```python
from build123d import *

# Parameters (mm, degrees)
SKETCH_1_W          = 63
SKETCH_1_H          = 15
SKETCH_1_R          = 1.1
SKETCH_1_R_2        = 1
SKETCH_1_R_3        = 1.5
SKETCH_1_R_4        = 2.6
EXTRUDE_1_DEPTH     = 2
SKETCH_2_R          = 1.4
EXTRUDE_2_DEPTH     = 2
SKETCH_3_R          = 3
CUT_EXTRUDE_1_DEPTH = 1.5
SKETCH_4_W          = 46
SKETCH_4_H          = 1.5
EXTRUDE_3_DEPTH     = 5
SKETCH_2_3_R        = 0.95
CUT_EXTRUDE_2_DEPTH = 1.5
CUT_EXTRUDE_3_DEPTH = 0.25
SKETCH_1_7_W        = 15
SKETCH_1_7_H        = 15
SKETCH_1_7_R        = 1.5
SKETCH_1_7_R_2      = 1.1
EXTRUDE_4_DEPTH     = 4
SKETCH_1_8_R        = 6
SKETCH_1_8_R_2      = 1.5
SKETCH_1_8_R_3      = 1.1
CUT_EXTRUDE_4_DEPTH = 2
CUT_EXTRUDE_5_DEPTH = 15
SKETCH_1_9_R        = 4
SKETCH_1_9_R_2      = 2.6
EXTRUDE_5_DEPTH     = 4


with BuildPart() as part:
    # 草图1 → 凸台-拉伸1 (new body)
    with BuildSketch(Plane(origin=(0, 0, 0), x_dir=(1, 0, 0), z_dir=(0, 1, 0))):
        Rectangle(SKETCH_1_W, SKETCH_1_H)
        with Locations(Location((-12.830127019, -2.5, 0), (0, 0, 270))):
            Circle(SKETCH_1_R, mode=Mode.SUBTRACT)
        with Locations(Location((3, 0, 0), (0, 0, 270))):
            Circle(SKETCH_1_R_2, mode=Mode.SUBTRACT)
        with Locations(Location((13, 0, 0), (0, 0, 270))):
            Circle(SKETCH_1_R_2, mode=Mode.SUBTRACT)
        with Locations(Location((-8.5, 0, 0), (0, 0, 270))):
            Circle(SKETCH_1_R_3, mode=Mode.SUBTRACT)
        with Locations(Location((-4.169872981, 2.5, 0), (0, 0, 270))):
            Circle(SKETCH_1_R, mode=Mode.SUBTRACT)
        with Locations(Location((8, 5, 0), (0, 0, 270))):
            Circle(SKETCH_1_R_2, mode=Mode.SUBTRACT)
        with Locations(Location((8, 0, 0), (0, 0, 270))):
            Circle(SKETCH_1_R_4, mode=Mode.SUBTRACT)
        with Locations(Location((24, 3.5, 0), (0, 0, 270))):
            Circle(SKETCH_1_R, mode=Mode.SUBTRACT)
        with Locations(Location((24, -3.5, 0), (0, 0, 270))):
            Circle(SKETCH_1_R, mode=Mode.SUBTRACT)
        with Locations(Location((20.5, 0, 0), (0, 0, 270))):
            Circle(SKETCH_1_R, mode=Mode.SUBTRACT)
        with Locations(Location((24, 0, 0), (0, 0, 270))):
            Circle(SKETCH_1_R_3, mode=Mode.SUBTRACT)
        with Locations(Location((27.5, 0, 0), (0, 0, 270))):
            Circle(SKETCH_1_R, mode=Mode.SUBTRACT)
    extrude(amount=EXTRUDE_1_DEPTH)

    # 草图2 → 凸台-拉伸2 (add)
    with BuildSketch(Plane.XY.offset(7.5)):
        with Locations(Location((-23.5, 0.6, 0), (0, 0, 205.376933525))):
            Circle(SKETCH_2_R)
        with Locations(Location((-8.5, 0.6, 0), (0, 0, 205.376933525))):
            Circle(SKETCH_2_R)
        with Locations(Location((6.5, 0.6, 0), (0, 0, 205.376933525))):
            Circle(SKETCH_2_R)
    extrude(amount=EXTRUDE_2_DEPTH)

    # 草图3 → 切除-拉伸1 (cut)
    with BuildSketch(Plane.XZ):
        with Locations(Location((-8.5, 0, 0), (0, 0, 270))):
            Circle(SKETCH_3_R)
    extrude(amount=-CUT_EXTRUDE_1_DEPTH, mode=Mode.SUBTRACT)

    # 草图4 → 凸台-拉伸3 (add)
    with BuildSketch(Plane.XZ):
        with Locations((-8.5, 6.75)):
            Rectangle(SKETCH_4_W, SKETCH_4_H)
    extrude(amount=EXTRUDE_3_DEPTH)

    # 草图2<3> → 切除-拉伸2 (cut)
    with BuildSketch(Plane.XY.offset(7.5)):
        with Locations((-23.5, -3.4)):
            Circle(SKETCH_2_3_R)
        with Locations((-8.5, -3.4)):
            Circle(SKETCH_2_3_R)
        with Locations((6.5, -3.4)):
            Circle(SKETCH_2_3_R)
    extrude(amount=-CUT_EXTRUDE_2_DEPTH, mode=Mode.SUBTRACT)

    # 草图5 → 切除-拉伸3 (cut)
    with BuildSketch(Plane(origin=(0, 0, 6), x_dir=(-1, 0, 0), z_dir=(0, 0, -1))):
        Polygon((22.403034489, -1.5), (24.596965511, -1.5), (25.693931023, -3.4), (24.596965511, -5.3), (22.403034489, -5.3), (21.306068977, -3.4), align=None)
        Polygon((6.306068977, -3.4), (7.403034489, -1.5), (9.596965511, -1.5), (10.693931023, -3.4), (9.596965511, -5.3), (7.403034489, -5.3), align=None)
        Polygon((-8.693931023, -3.4), (-7.596965511, -1.5), (-5.403034489, -1.5), (-4.306068977, -3.4), (-5.403034489, -5.3), (-7.596965511, -5.3), align=None)
    extrude(amount=-CUT_EXTRUDE_3_DEPTH, mode=Mode.SUBTRACT)

    # 草图1<7> → 凸台-拉伸4 (add)
    with BuildSketch(Plane(origin=(0, 0, 0), x_dir=(1, 0, 0), z_dir=(0, 1, 0))):
        with Locations((24, 0)):
            Rectangle(SKETCH_1_7_W, SKETCH_1_7_H)
        with Locations(Location((24, 0, 0), (0, 0, 270))):
            Circle(SKETCH_1_7_R, mode=Mode.SUBTRACT)
        with Locations(Location((27.5, 0, 0), (0, 0, 270))):
            Circle(SKETCH_1_7_R_2, mode=Mode.SUBTRACT)
        with Locations(Location((24, -3.5, 0), (0, 0, 270))):
            Circle(SKETCH_1_7_R_2, mode=Mode.SUBTRACT)
        with Locations(Location((20.5, 0, 0), (0, 0, 270))):
            Circle(SKETCH_1_7_R_2, mode=Mode.SUBTRACT)
        with Locations(Location((24, 3.5, 0), (0, 0, 270))):
            Circle(SKETCH_1_7_R_2, mode=Mode.SUBTRACT)
    extrude(amount=EXTRUDE_4_DEPTH)

    # 草图1<8> → 切除-拉伸4 (cut)
    with BuildSketch(Plane(origin=(0, 0, 0), x_dir=(1, 0, 0), z_dir=(0, 1, 0))):
        with Locations(Location((24, 0, 0), (0, 0, 270))):
            Circle(SKETCH_1_8_R)
        with Locations(Location((24, 0, 0), (0, 0, 270))):
            Circle(SKETCH_1_8_R_2, mode=Mode.SUBTRACT)
        with Locations(Location((27.5, 0, 0), (0, 0, 270))):
            Circle(SKETCH_1_8_R_3, mode=Mode.SUBTRACT)
        with Locations(Location((24, -3.5, 0), (0, 0, 270))):
            Circle(SKETCH_1_8_R_3, mode=Mode.SUBTRACT)
        with Locations(Location((20.5, 0, 0), (0, 0, 270))):
            Circle(SKETCH_1_8_R_3, mode=Mode.SUBTRACT)
        with Locations(Location((24, 3.5, 0), (0, 0, 270))):
            Circle(SKETCH_1_8_R_3, mode=Mode.SUBTRACT)
    extrude(amount=CUT_EXTRUDE_4_DEPTH, mode=Mode.SUBTRACT)

    # 草图6 → 切除-拉伸5 (cut)
    with BuildSketch(Plane(origin=(0, 0, -7.5), x_dir=(-1, 0, 0), z_dir=(0, 0, -1))):
        Polygon((-16.5, 2), (-18.5, 4), (-16.5, 4), align=None)
    extrude(amount=-CUT_EXTRUDE_5_DEPTH, mode=Mode.SUBTRACT)

    # 草图1<9> → 凸台-拉伸5 (add)
    with BuildSketch(Plane(origin=(0, 0, 0), x_dir=(1, 0, 0), z_dir=(0, 1, 0))):
        with Locations(Location((8, 0, 0), (0, 0, 89.999818815))):
            Circle(SKETCH_1_9_R)
        with Locations(Location((8, 0, 0), (0, 0, 270))):
            Circle(SKETCH_1_9_R_2, mode=Mode.SUBTRACT)
    extrude(amount=EXTRUDE_5_DEPTH)


solid = part.part
```
Geometry: final body of the model. Coordinates: model frame, mm. A direction names the side the tool comes from. Give positions to 0.01 mm unless a question says otherwise; leave off trailing zeros. Loops run counter-clockwise (first coordinate to the right, second up) from the corner with the lowest first, then second, coordinate; pieces in that order, holes last. Notation, with made-up numbers: (-30.75, 19) -> (28.25, 19) arc R22 cw to (28.25, 40) -> close; hole circle Ø9 at (14.5, 81.5). An arc over 180 degrees is marked (long way). Use CSV: the item, a comma, the result in double quotes.
(1) Cut plane D-D (x = -27.5). Output: boundary loops of the cut face in (y, z).
From the geometry:
outline,"(-5, 6) -> (0, 6) -> (0, -7.5) -> (2, -7.5) -> (2, 7.5) -> (-5, 7.5) -> close"
(2) Access query for faces 4 (the face through (6, -2, 6.25)), 5 (the face through (-24.9, 0.53, 8.49)), 6 (the face through (6.6, 1.5, -7.5)), 7 (the face through (22.8, 2, 1.2)). Directions: +Z, -Z, +X, -X, +Y, -Y. A direction counts if a zero-diameter tool reaches every point of the face in a straight line with its end or side. Return the directions, or none.
From the geometry:
face 4,"-Z"
face 5,"+Z"
face 6,"-Z, +X, -X, +Y, -Y"
face 7,"-Y"
(3) Cut plane A-A (x = 24). Output: boundary loops of the cut face in (y, z), plus the area to 3 significant figures.
From the geometry:
outline,"(0, -7.5) -> (4, -7.5) -> (4, -4.6) -> (2, -4.6) -> (2, -6) -> (0, -6) -> close; (0, 6) -> (2, 6) -> (2, 4.6) -> (4, 4.6) -> (4, 7.5) -> (0, 7.5) -> close; (2, -2.4) -> (4, -2.4) -> (4, -1.5) -> (2, -1.5) -> close; (2, 1.5) -> (4, 1.5) -> (4, 2.4) -> (2, 2.4) -> close"
area,"21.2 mm^2"
(4) Cut plane B-B (x = 13). Output: boundary loops of the cut face in (y, z).
From the geometry:
outline,"(-5, 6) -> (0, 6) -> (0, 1) -> (2, 1) -> (2, 7.5) -> (-5, 7.5) -> close; (0, -7.5) -> (2, -7.5) -> (2, -1) -> (0, -1) -> close"
(5) Ray query, line 1 along X through (y, z) = (1.9, 0); line 2 along X through (y, z) = (0.8, 0); line 3 along Y through (x, z) = (6.5, 6.6). Return the intervals inside material, ascending. Write a range as [from, to].
From the geometry:
line 1,"[-31.5, -10], [-7, 2], [4, 5.4], [10.6, 12], [14, 18], [30, 31.5]"
line 2,"[-31.5, -11.5], [-5.5, 2], [4, 5.4], [10.6, 12], [14, 18], [30, 31.5]"
line 3,"[-5, -4.35], [-2.45, 2]"
(6) Cut plane C-C (y = 0.6). Count the separate pieces of the cut face and the enclosed holes in it, plus the area to 3 significant figures.
From the geometry:
separate pieces,"1"
enclosed holes,"8"
area,"782 mm^2"
(7) First-contact query: P1, Ø9.5, axis at x = 21, z = 2.5, coming from the -Y side; P2, Ø0.8, axis at y = -2.5, z = 7, coming from the +X side; P3, Ø1.5, axis at x = -22.5, y = -2.5, coming from the -Z side; P4, Ø10, axis at x = 1.5, z = 1.5, coming from the -Y side. Flat tips, straight axial feed; report the tip coordinate or a pass-through.
From the geometry:
P1,"y = 0"
P2,"x = 14.5"
P3,"z = 6"
P4,"y = -5"
(8) Pull-direction query (X, two-part tool) for faces 1 (the face through (-7, 0, -3)), 2 (the face through (-31.5, 1, 2)), 3 (the face through (-3.84, 0.99, -1.45)); classes: released by +X, released by -X, zero draft, split by the parting line, or undercut.
From the geometry:
face 1,"zero draft"
face 2,"released by -X"
face 3,"undercut"
